For this review, use the dimensioned drawing (mm, ordinates from the lowest corner) and the shaded views. Coordinates: 2 decimals unless noted, no trailing zeros. Write each loop counter-clockwise with the first axis right and the second up, starting at its lowest first coordinate (ties: lowest second). Pieces come first, ordered by that corner, then holes. Notation, with made-up numbers: M 64,-9 L 69,-9 A20 ccw 69,7 Z; hole C 43.5,78.25 d2. An arc over 180 degrees is marked long. One line per question, with ' | ' between items.
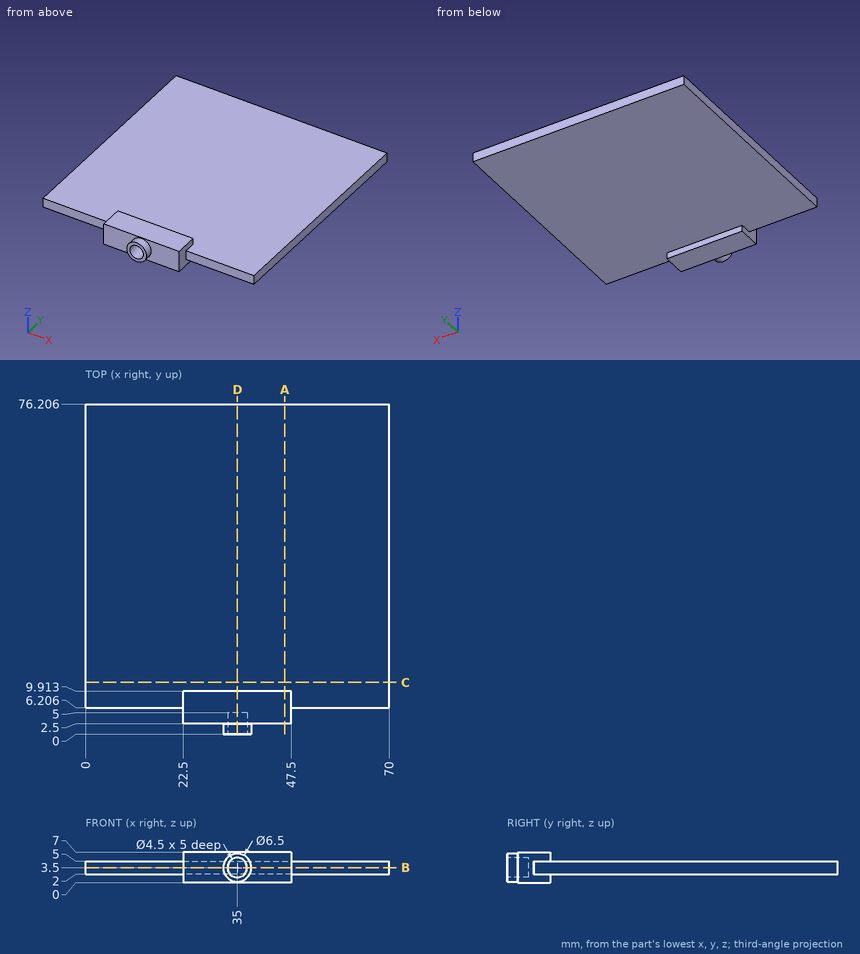
1) Insertion check: pin 1 Ø2 at (x, z) = (32.5, 5) entering from -Y; pin 2 Ø1.5 at (x, z) = (16.5, 1) entering from +Y; pin 3 Ø0.9 at (x, z) = (13.5, 3.5) entering from -Y; pin 4 Ø1.6 at (x, z) = (32, 1) entering from +Y. Each pin has a flat end and moves straight along its axis. Give the tip position at first contact, or say it passes through.
Responses:
pin 1: y = 0 | pin 2: through | pin 3: y = 6.21 | pin 4: y = 9.91
2) We need section B-B on z = 3.5. State the section outline as (x, y) points.
Responses:
outline: M 0,6.21 L 22.5,6.21 L 22.5,2.5 L 31.75,2.5 L 31.75,0 L 32.75,0 L 32.75,5 L 37.25,5 L 37.25,0 L 38.25,0 L 38.25,2.5 L 47.5,2.5 L 47.5,6.21 L 70,6.21 L 70,76.21 L 0,76.21 Z
3) We need section A-A on x = 46. State the section outline as (y, z) points, then the cut area to 3 significant figures.
Responses:
outline: M 2.5,0 L 9.91,0 L 9.91,2 L 76.21,2 L 76.21,5 L 9.91,5 L 9.91,7 L 2.5,7 Z | area: 251 mm^2
4) We need section D-D on x = 35. State the section outline as (y, z) points.
Responses:
outline: M 0,0.25 L 2.5,0.25 L 2.5,0 L 9.91,0 L 9.91,2 L 76.21,2 L 76.21,5 L 9.91,5 L 9.91,7 L 2.5,7 L 2.5,6.75 L 0,6.75 L 0,5.75 L 5,5.75 L 5,1.25 L 0,1.25 Z
5) We need section C-C on y = 12. State the section outline as (x, z) points.
Responses:
outline: M 0,2 L 70,2 L 70,5 L 0,5 Z
6) To check wall thickness, follow line 1 along X through (y, z) = (2.4, 3.5); line 2 along X through (y, z) = (3.2, 3.5); line 3 along Z through (x, y) = (11, 28). State the ranges of each line that lie inside material, in increasing order. Write a range as [from, to].
Responses:
line 1: [31.75, 32.75], [37.25, 38.25] | line 2: [22.5, 32.75], [37.25, 47.5] | line 3: [2, 5]
